from build123d import *

# Parameters (mm, degrees)
F0_W     = 66.714566201
F0_H     = 88.7944847345
F1_DEPTH = 25.4
F2_R     = 5.08
F3_R     = 2.1888893323
F4_DEPTH = 1.27
F5_R     = 0.63499


# Not quite as in the source:
# - a fillet or chamfer is up to 0.001 mm smaller than in the source, because OpenCascade refuses the exact size


with BuildPart() as f1:
    # F0 (on Front) → F1 (new body)
    with BuildSketch(Plane.XZ):
        with Locations((0.118708238, -3.5612769425)):
            Rectangle(F0_W, F0_H)
    extrude(amount=F1_DEPTH)

    # F2
    f2_edges = [f1.edges().sort_by_distance(p)[0] for p in [
        (33.475991, -25.4, -3.561277),
        (0.118708, -25.4, -47.958519),
        (33.475991, -12.7, -47.958519),
        (33.475991, -12.7, 40.835965),
        (33.475991, 0, -3.561277),
        (0.118708, -25.4, 40.835965),
        (-33.238575, -12.7, 40.835965),
        (-33.238575, -12.7, -47.958519),
        (-33.238575, 0, -3.561277),
        (-33.238575, -25.4, -3.561277),
        (0.118708, 0, 40.835965),
        (0.118708, 0, -47.958519),
    ]]
    fillet(f2_edges, radius=F2_R)

    # F3 (on face) → F4 (join)
    with BuildSketch(Plane(origin=(0, 0, -47.9585193098), x_dir=(1, 0, 0), z_dir=(0, 0, -1))):
        with Locations((-20.655401051, 16.3818709552)):
            Circle(F3_R)
    extrude(amount=F4_DEPTH)

    # F5 (radius 0.635 in the source; OpenCascade refuses exactly that, so slightly less here)
    f5_edges = [f1.edges().sort_by_distance(p)[0] for p in [
        (-22.84429, -16.381871, -49.228519),
        (-22.84429, -16.381871, -47.958519),
        (-18.466512, -16.381871, -48.593519),
    ]]
    fillet(f5_edges, radius=F5_R)


solid = f1.part
Work out the finished part from the listing and answer in its coordinate system (mm). Coordinates: 2 decimals unless noted, no trailing zeros. Loops run counter-clockwise (first coordinate to the right, second up) from the corner with the lowest first, then second, coordinate; pieces in that order, holes last. Notation, with made-up numbers: (17, -10.5) -> (40, -10.5) arc R28 cw to (40, 24.5) -> close; hole circle Ø3 at (-40, 65.25). An arc over 180 degrees is marked (long way). Write each question's results on one line, items separated by ' | '. Start each with the question number.
1) Consider line 1 along Z through (x, y) = (6, -12); line 2 along X through (y, z) = (-5, 27.5); line 3 along Y through (x, z) = (-23, 36). Determine where each line is inside the solid, lowest interval first.
2) Find section B-B on x = 19.5. Determine the outline of the cut face in (y, z), then the cut area to 3 significant figures.
3) Flat-ended cylindrical pins translate along their axes: P1, Ø4, axis at y = -21.5, z = -24, coming from the +X side; P2, Ø1, axis at y = -3.5, z = -34.5, coming from the -X side. Find the tip coordinate at first contact, or state that the pin passes through.
4) Find section A-A on y = -10.5. Determine the outline of the cut face in (x, z), then the cut area to 3 significant figures.
Response values:
1) line 1: z = -47.96 to 40.84 | line 2: x = -33.24 to 33.48 | line 3: y = -25.39 to -0.01
2) outline: (-25.4, -42.88) arc R5.08 ccw to (-20.32, -47.96) -> (-5.08, -47.96) arc R5.08 ccw to (0, -42.88) -> (0, 35.76) arc R5.08 ccw to (-5.08, 40.84) -> (-20.32, 40.84) arc R5.08 ccw to (-25.4, 35.76) -> close | area: 2,230 mm^2
3) P1: stops at x = 33.48 | P2: stops at x = -33.12
4) outline: (-33.24, -42.88) arc R5.08 ccw to (-28.16, -47.96) -> (28.4, -47.96) arc R5.08 ccw to (33.48, -42.88) -> (33.48, 35.76) arc R5.08 ccw to (28.4, 40.84) -> (-28.16, 40.84) arc R5.08 ccw to (-33.24, 35.76) -> close | area: 5,900 mm^2
